Geometry: final body of the model. Coordinates: model frame, mm. Give positions to 0.01 mm unless a question says otherwise; leave off trailing zeros. Write each loop counter-clockwise with the first axis right and the second up, starting at its lowest first coordinate (ties: lowest second). Pieces come first, ordered by that corner, then holes. Notation, with made-up numbers: (48.25, -38) - (93.25, -38) arc R9 ccw to (93.25, -22) - close; hole circle Ø1 at (24.5, 73). An arc over 180 degrees is marked (long way). Use CSV: the item, a comma, the result in double quotes. Start each with the question number.
(1) First-contact query: pin 1 Ø1.5 at (y, z) = (7, 0) entering from +X; pin 2 Ø1.5 at (y, z) = (6.5, 1.5) entering from -X. Flat tips, straight axial feed; report the tip coordinate or a pass-through.
(2) Section A-A on y = 5.75. Output: boundary loops of the cut face in (x, z).
(3) Section B-B on x = 6.75. Output: boundary loops of the cut face in (y, z) (3 decimals).
(4) Line query: probe 1 along Z at (x, y) = (0, 6); probe 2 along Z at (x, y) = (3.25, 4.75). Output: solid intervals per line, ascending. Write a range as [from, to].
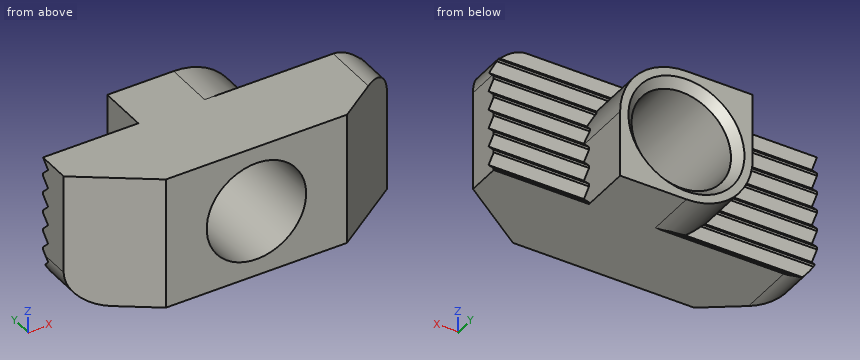
Autodesk Inventor part; units mm, degrees
ref_plane "YZ Plane" through (0, 0, 0) normal (1, 0, 0) x (0, 1, 0)
ref_plane "XZ Plane" through (0, 0, 0) normal (0, 1, 0) x (-1, 0, 0)
ref_plane "XY Plane" through (0, 0, 0) normal (0, 0, 1) x (1, 0, 0)
sketch "Skizze3" plane through (0, 0, 0) normal (0, 0, 1) x (1, 0, 0)
  line L0 (0, 0) -> (5.4656, 0)
  line L1 (5.4656, 0) -> (9.75, 3)
  line L2 (9.75, 3) -> (9.75, 5)
  line L3 (9.75, 5) -> (0, 5)
  line L4 (0, 6) -> (0, -1) construction
  line L5 (0, 0) -> (-5.4656, 0)
  line L6 (-5.4656, 0) -> (-9.75, 3)
  line L7 (-9.75, 3) -> (-9.75, 5)
  line L8 (-9.75, 5) -> (0, 5)
  dimension "d6" = 9.75
  dimension "d8" = 5
  dimension "d9" = 3
  dimension "d10" = 145
extrude "Extrusion2" add sketch "Skizze3" along normal mid plane 8
sketch "Skizze4" plane through (-9.75, 5, 4) normal (0, 1, 0) x (1, 0, 0)
  line L0 (0, 8) -> (0, 0)
  line L1 (19.5, 0) -> (0, 0)
  line L2 (19.5, 8) -> (19.5, 0)
  line L3 (0, 8) -> (19.5, 8)
  circle A0 centre (9.75, 4) radius 3
  line L4 (5.75, 8) -> (13.75, 8)
  line L5 (13.75, 8) -> (13.75, 0)
  line L6 (13.75, 0) -> (5.75, 0)
  line L7 (5.75, 0) -> (5.75, 8)
  line L8 (5.75, 8) -> (13.75, 0) construction
  line L9 (13.75, 8) -> (5.75, 0) construction
  line L10 (0, 8) -> (19.5, 8)
  arc A1 (9.75, 8) -> (5.75, 4) centre (9.75, 4) ccw
  arc A2 (9.75, 0) -> (13.75, 4) centre (9.75, 4) ccw
  point P0 (9.75, 0)
  dimension "d13" = 6
  dimension "d14" = 8
  dimension "d15" = 8
extrude "Extrusion3" add sketch "Skizze4" along normal blind 3 and the other way blind 5 separate body contours L7 A1 L3 L5 A2 L1
sketch "Skizze5" plane through (9.75, 3, 4) normal (1, 0, 0) x (0, 0, -1)
  line L0 (8, 2) -> (0, 2)
  line L1 (0, 0) -> (0, 2)
  line L2 (8, 0) -> (0, 0)
  line L3 (8, 2) -> (8, 0)
  line L4 (0, 0) -> (0, 2)
  line L5 (0, 2) -> (0.495, 1.505)
  line L6 (0.495, 1.505) -> (0.9899, 2)
  line L7 (8, 2) -> (0, 2)
  line L8 (1.15, 2) -> (1.645, 1.505)
  line L9 (1.645, 1.505) -> (2.1399, 2)
  line L10 (2.3, 2) -> (2.795, 1.505)
  line L11 (2.795, 1.505) -> (3.2899, 2)
  line L12 (3.45, 2) -> (3.945, 1.505)
  line L13 (3.945, 1.505) -> (4.4399, 2)
  line L14 (4.6, 2) -> (5.095, 1.505)
  line L15 (5.095, 1.505) -> (5.5899, 2)
  line L16 (5.75, 2) -> (6.245, 1.505)
  line L17 (6.245, 1.505) -> (6.7399, 2)
  line L18 (6.9, 2) -> (7.395, 1.505)
  line L19 (7.395, 1.505) -> (7.8899, 2)
  point P0 (4, -3)
  dimension "d21" = 0.7
  dimension "d24" = 1.15
extrude "Extrusion4" cut sketch "Skizze5" against normal up to surface (19.5 mm away) contours L19 L18 L0 | L17 L16 L0 | L0 L6 L5 | L15 L14 L0 | L0 L9 L8 | L13 L12 L0 | L0 L11 L10 bodies 1
extrude "Extrusion5" cut sketch "Skizze4" against normal blind 10 contours A0 bodies 1
chamfer "Fase2" distance 0.5 angle 45 1 edges at (-3, 8, 0)
combine bodies "Kombinieren1" operation type add bodies to combine 1 2
fillet "Rundung1" radius 2 2 edges at (9.75, 4, 4) (-9.75, 4, -4)
properties part number "T-NUT - DropIn 4040 SERIES - M6"
Check values:
1,pin 1,"stops at x = 4"
1,pin 2,"stops at x = -4"
2,outline,"(-4, 0) arc R4 ccw to (0, -4) - (4, -4) - (4, 0) arc R4 ccw to (0, 4) - (-4, 4) - close; hole circle Ø6 at (0, 0)"
3,outline,"(0.899, -4) - (5, -4) - (5, -3.89) - (4.505, -3.395) - (5, -2.9) - (5, -2.74) - (4.505, -2.245) - (5, -1.75) - (5, -1.59) - (4.505, -1.095) - (5, -0.6) - (5, -0.44) - (4.505, 0.055) - (5, 0.55) - (5, 0.71) - (4.505, 1.205) - (5, 1.7) - (5, 1.86) - (4.505, 2.355) - (5, 2.85) - (5, 3.01) - (4.505, 3.505) - (5, 4) - (0.899, 4) - close"
4,probe 1,"z = [-4, -3], [3, 4]"
4,probe 2,"z = [-4, 2.33], [2.6, 3.26], [3.75, 4]"
